The drawing under review shows one solid part. Ordinate dimensions are in mm from its lowest x, y, z. Give positions to 0.01 mm unless a question says otherwise; leave off trailing zeros. Loops run counter-clockwise (first coordinate to the right, second up) from the corner with the lowest first, then second, coordinate; pieces in that order, holes last. Notation, with made-up numbers: (6.5, 56) - (44.5, 56) arc R32 cw to (44.5, 83) - close; hole circle Ø8 at (80.5, -7). An arc over 180 degrees is marked (long way). One line per item, written item: value. Start each with the question number.
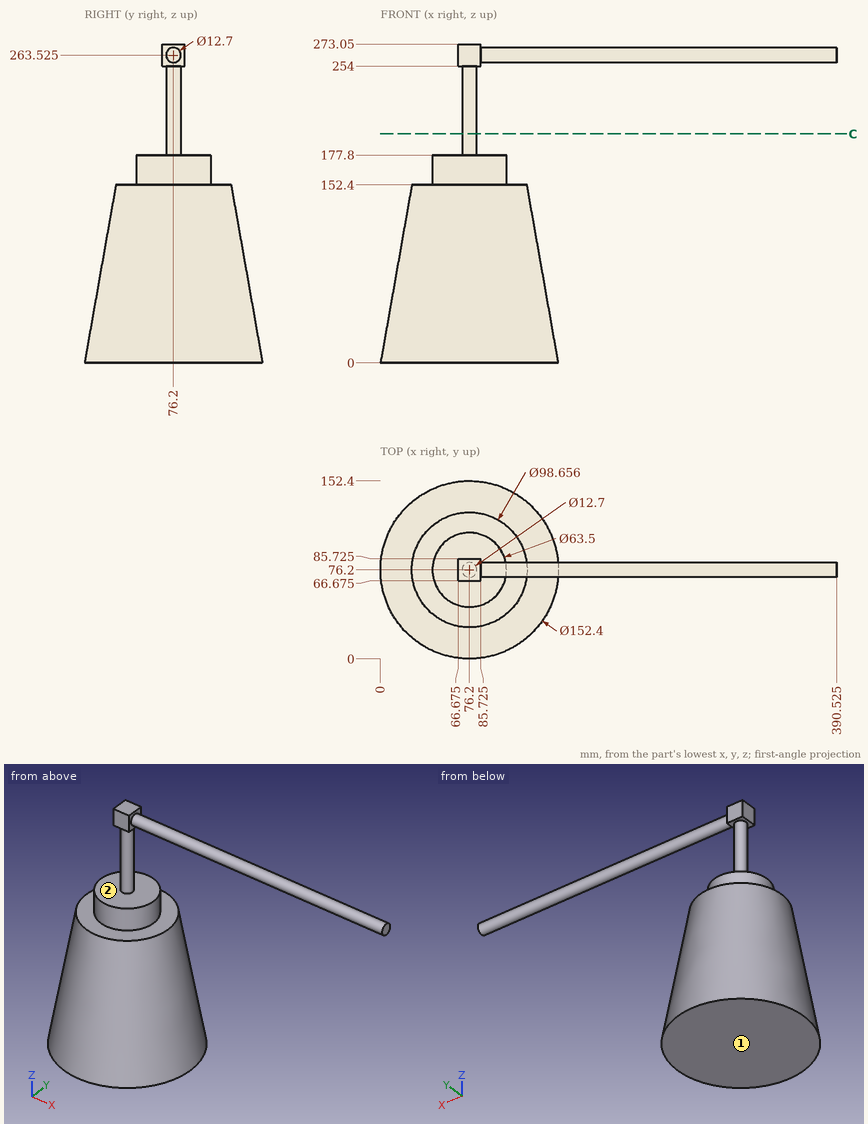
(1) For pin 1 Ø10 at (x, y) = (334.5, 84) entering from +Z (1 decimal); pin 2 Ø9.5 at (y, z) = (80.5, 261) entering from -X (3 decimals); pin 3 Ø8 at (y, z) = (102, 162.5) entering from +X, all flat-tipped, find the tip position at first contact; note any pin that passes through.
(2) Draft analysis for pull direction Z (two halves, no side actions). For the marked faces 1 and 2, state which applies: pulls with the +Z half, pulls with the -Z half, needs draft (parallel to the pull), parting line crosses it, or undercut.
(3) To check wall thickness, follow L1, parallel to Z at x = 259, y = 77 (1 decimal); L2, parallel to X at y = 28.5, z = 45.5; L3, parallel to X at y = 111, z = 113 (1 decimal). State the ranges of each line that lie inside material, in increasing order. Write a range as from..to.
(4) Take a section at C-C on z = 196. State the section outline as (x, y) points.
Here are the results:
1. pin 1: z = 269.2
1. pin 2: x = 66.675
1. pin 3: x = 99.28
2. face 1: pulls with the -Z half
2. face 2: undercut
3. L1: 257.2..269.8
3. L2: 27.49..124.91
3. L3: 32..120.4
4. outline: circle Ø12.7 at (76.2, 76.2)
